from build123d import *

# Parameters (mm, degrees)
SKETCH2_W               = 25
SKETCH2_H               = 9
BOSS_EXTRUDE3_DEPTH     = 6
SKETCH3_R               = 2.55
CUT_EXTRUDE1_DEPTH      = 5
CUT_EXTRUDE2_DEPTH      = 28.239676944
CUT_EXTRUDE2_DEPTH_BACK = 28.239676944
SKETCH4_R               = 1.5
SKETCH5_R               = 1.5
CUT_EXTRUDE3_DEPTH      = 4.5
CUT_EXTRUDE4_DEPTH      = 28.239676944
FILLET2_R               = 0.4
SKETCH8_R               = 1
CUT_EXTRUDE5_DEPTH      = 28.239676944
CUT_EXTRUDE7_DEPTH      = 10


with BuildPart() as part:
    # Sketch2 → Boss-Extrude3 (new body)
    with BuildSketch(Plane(origin=(0, 0, 0), x_dir=(1, 0, 0), z_dir=(0, 1, 0))):
        with Locations((12.5, 4.5)):
            Rectangle(SKETCH2_W, SKETCH2_H)
    extrude(amount=BOSS_EXTRUDE3_DEPTH)

    # Sketch3 → Cut-Extrude1 (cut)
    with BuildSketch(Plane(origin=(0, 6, 0), x_dir=(1, 0, 0), z_dir=(0, 1, 0))):
        with Locations(Location((4.5, 4.5, 0), (0, 0, 270))):
            Circle(SKETCH3_R)
    extrude(amount=-CUT_EXTRUDE1_DEPTH, mode=Mode.SUBTRACT)

    # Sketch4 → Cut-Extrude2 (cut, two sides: drawn at the far end of the back side and taken through both)
    with BuildSketch(Plane(origin=(0, 6, 0), x_dir=(1, 0, 0), z_dir=(0, 1, 0)).offset(-CUT_EXTRUDE2_DEPTH_BACK)):
        with Locations(Location((22.25, 4.5, 0), (0, 0, 270))):
            Circle(SKETCH4_R)
    extrude(amount=CUT_EXTRUDE2_DEPTH + CUT_EXTRUDE2_DEPTH_BACK, mode=Mode.SUBTRACT)

    # Sketch5 → Cut-Extrude3 (cut)
    with BuildSketch(Plane(origin=(0, 6, 0), x_dir=(1, 0, 0), z_dir=(0, 1, 0))):
        with BuildLine():
            Line((25, 9), (4.5, 9))
            ThreePointArc((4.5, 9), (7.681980515, 7.681980515), (9, 4.5))
            ThreePointArc((9, 4.5), (7.681980515, 1.318019485), (4.5, 0))
            Line((4.5, 0), (25, 0))
            Line((25, 0), (25, 9))
        make_face()
        with Locations(Location((22.25, 4.5, 0), (0, 0, 270))):
            Circle(SKETCH5_R, mode=Mode.SUBTRACT)
    extrude(amount=-CUT_EXTRUDE3_DEPTH, mode=Mode.SUBTRACT)

    # Sketch6 → Cut-Extrude4 (cut, through all)
    with BuildSketch(Plane(origin=(0, 6, 0), x_dir=(1, 0, 0), z_dir=(0, 1, 0))):
        with BuildLine():
            ThreePointArc((0, 4.5), (1.318019485, 7.681980515), (4.5, 9))
            Line((4.5, 9), (0, 9))
            Line((0, 9), (0, 4.5))
        make_face()
        with BuildLine():
            ThreePointArc((4.5, 0), (1.318019485, 1.318019485), (0, 4.5))
            Line((0, 4.5), (0, 0))
            Line((0, 0), (4.5, 0))
        make_face()
    extrude(amount=-CUT_EXTRUDE4_DEPTH, mode=Mode.SUBTRACT)

    # Fillet2
    fillet2_edges = [part.edges().sort_by_distance(p)[0] for p in [
        (4.5, 6, -7.05),
    ]]
    fillet(fillet2_edges, radius=FILLET2_R)

    # Sketch8 → Cut-Extrude5 (cut, through all)
    with BuildSketch(Plane.XZ):
        with Locations(Location((4.5, -4.5, 0), (0, 0, 270))):
            Circle(SKETCH8_R)
    extrude(amount=-CUT_EXTRUDE5_DEPTH, mode=Mode.SUBTRACT)

    # Sketch9 → Cut-Extrude7 (cut)
    with BuildSketch(Plane(origin=(0, 1.5, 0), x_dir=(1, 0, 0), z_dir=(0, 1, 0))):
        with BuildLine():
            Line((25, 9), (4.5, 9))
            ThreePointArc((4.5, 9), (6.368244423, 8.593856712), (7.899255542, 7.448739011))
            ThreePointArc((7.899255542, 7.448739011), (11.227526502, 5.656546092), (15, 5.416157335))
            Line((15, 5.416157335), (21.94811323, 6.477084818))
            ThreePointArc((21.94811323, 6.477084818), (24.25, 4.499999978), (21.948113186, 2.522915189))
            Line((21.948113186, 2.522915189), (15, 3.583842665))
            ThreePointArc((15, 3.583842665), (11.227526502, 3.343453908), (7.899255542, 1.551260989))
            ThreePointArc((7.899255542, 1.551260989), (6.368244423, 0.406143288), (4.5, 0))
            Line((4.5, 0), (25, 0))
            Line((25, 0), (25, 9))
        make_face()
    extrude(amount=-CUT_EXTRUDE7_DEPTH, mode=Mode.SUBTRACT)


solid = part.part
Input: part model. Units: mm. Frame: model coordinates. A direction names the side the tool comes from. Give positions to 0.01 mm unless a question says otherwise; leave off trailing zeros. Loops run counter-clockwise (first coordinate to the right, second up) from the corner with the lowest first, then second, coordinate; pieces in that order, holes last. Notation, with made-up numbers: (-24, 71.25) - (18, 71.25) arc R25 ccw to (18, 90.25) - close; hole circle Ø10 at (52, 20.25). An arc over 180 degrees is marked (long way). Use CSV: the item, a comma, the result in double quotes. Start each with the question number.
Item 1: Mould query, pull axis X, two halves, no side actions, for faces 6 (the flat face through (9, 0, -5)), 7 (the cylindrical face through (23.737, 0.739, -4.695)). Classes: pulls with the +X half, pulls with the -X half, needs draft (parallel to the pull), parting line crosses it, or undercut.
Item 2: Line query: line 1 (X direction, y = 0.7, z = -4.5); line 2 (Z direction, x = 22.25, y = 1.1); line 3 (X direction, y = 3.75, z = -6.25). Output: solid intervals per line, ascending.
Item 3: Section A-A on x = 22.25. Return loops of the section in (y, z), then the cut area to 3 significant figures.
Item 4: Contact query for flat-ended pins moving along their axis: P1, Ø4, axis at x = 4, z = -4.5, coming from the +Y side; P2, Ø1, axis at y = 4, z = -1, coming from the +X side; P3, Ø1.8, axis at x = 20, z = -5, coming from the +Y side. Output: stop coordinate, or through.
Item 5: Section D-D on z = -8. Return loops of the section in (x, y).
Item 6: Section C-C on y = 3.2. Return loops of the section in (x, z).
Item 7: Section B-B on y = 0.6. Return loops of the section in (x, z), then the cut area to 3 significant figures.
Item 8: Reachability of faces 1 (the flat face through (18.43, 0.76, -5.94)), 2 (the flat face through (18.523, 0.76, -3.046)), 3 (the flat face through (5, 1, -3)), 4 (the flat face through (3.4, 6, -1.6)), 5 (the cylindrical face through (5.176, 0.493, -3.763)) from +Z, -Z, +X, -X, +Y, -Y: full face, straight path, thin tool, end or side. Return the list, or none.
Ans:
1,face 6,"needs draft"
1,face 7,"undercut"
2,line 1,"x = 0 to 3.5, 5.5 to 20.75, 23.75 to 24.25"
2,line 2,"z = -6.5 to -6, -3 to -2.5"
2,line 3,"x = 0.35 to 2.65, 6.35 to 8.65"
3,outline,"(0, -6.5) - (1.5, -6.5) - (1.5, -6) - (0, -6) - close; (0, -3) - (1.5, -3) - (1.5, -2.5) - (0, -2.5) - close"
3,area,"1.50 mm2"
4,P1,"stops at y = 1"
4,P2,"stops at x = 7.85"
4,P3,"stops at y = 1.5"
5,outline,"(1.67, 0) - (7.33, 0) - (7.33, 6) - (1.67, 6) - close"
6,outline,"circle Ø9 at (4.5, -4.5); hole circle Ø5.1 at (4.5, -4.5)"
7,outline,"(7.9, -7.45) arc R8.85 cw to (15, -5.42) - (21.95, -6.48) arc R2 ccw (long way) to (21.95, -2.52) - (15, -3.58) arc R8.85 cw to (7.9, -1.55) arc R4.5 ccw (long way) to start; hole circle Ø2 at (4.5, -4.5); hole circle Ø3 at (22.25, -4.5)"
7,area,"96.0 mm2"
8,face 1,"-Z, +Y, -Y"
8,face 2,"+Z, +Y, -Y"
8,face 3,"+Y"
8,face 4,"+Z, -Z, +X, -X, +Y"
8,face 5,"+Y, -Y"
